Build history of the part. All positions in model axes, mm. A direction names the side the tool comes from. Coordinates: 2 decimals unless noted, no trailing zeros. Order: outer loops, then holes, each group sorted by start corner. A loop starts at its lowest first (then second) coordinate and runs counter-clockwise, first axis right, second up. Notation, with made-up numbers: (75.25, 17.25) - (123.25, 17.25) arc R19 ccw to (123.25, 43.25) - close; hole circle Ø10 at (57, 52). An arc over 180 degrees is marked (long way). Answer as CSV lines item,"result". Start each with the question number.
from build123d import *

# Parameters (mm, degrees)
SKETCH1_W                               = 96
SKETCH1_H                               = 64
BOSS_EXTRUDE1_DEPTH                     = 20
CBORE_FOR_M6_HEX_HEAD_BOLT1_D           = 6.4
CBORE_FOR_M6_HEX_HEAD_BOLT1_CBORE_D     = 14.547
CBORE_FOR_M6_HEX_HEAD_BOLT1_CBORE_DEPTH = 4
BOSS_EXTRUDE3_DEPTH                     = 60
CUT_EXTRUDE1_DEPTH                      = 12
SKETCH14_R                              = 26
SKETCH14_R_2                            = 16
BOSS_EXTRUDE4_DEPTH                     = 32
BOSS_EXTRUDE8_START                     = -12
BOSS_EXTRUDE8_DEPTH                     = 12
SKETCH17_R                              = 16
CUT_EXTRUDE2_DEPTH                      = 198.440406876


with BuildPart() as part:
    # Sketch1 → Boss-Extrude1 (new body)
    with BuildSketch(Plane(origin=(0, 0, 0), x_dir=(0, 0, -1), z_dir=(1, 0, 0))):
        Rectangle(SKETCH1_W, SKETCH1_H)
    extrude(amount=BOSS_EXTRUDE1_DEPTH)

    # CBORE for M6 Hex Head Bolt1 (through all)
    with Locations(Plane(origin=(20, 0, -30), x_dir=(0, 0, 1), z_dir=(1, 0, 0))):
        with Locations((0, 0)):
            cbore_for_m6_hex_head_bolt1 = CounterBoreHole(CBORE_FOR_M6_HEX_HEAD_BOLT1_D / 2, CBORE_FOR_M6_HEX_HEAD_BOLT1_CBORE_D / 2, CBORE_FOR_M6_HEX_HEAD_BOLT1_CBORE_DEPTH)

    # Mirror1: CBORE for M6 Hex Head Bolt1 across plane
    add(cbore_for_m6_hex_head_bolt1.mirror(Plane.XY), mode=Mode.SUBTRACT)

    # Sketch11 → Boss-Extrude3 (add)
    with BuildSketch(Plane(origin=(0, 0, -30), x_dir=(0, -1, 0), z_dir=(0, 0, 1))):
        with BuildLine():
            ThreePointArc((20, 97.56139982), (22.055252622, 107.893852494), (27.908116908, 116.653282912))
            Line((27.908116908, 116.653282912), (75.840620434, 164.585786438))
            Line((75.840620434, 164.585786438), (84.325901808, 156.100505063))
            Line((84.325901808, 156.100505063), (36.393398282, 108.168001538))
            ThreePointArc((36.393398282, 108.168001538), (33.141807012, 103.301651305), (32, 97.56139982))
            Line((32, 97.56139982), (32, 20))
            Line((32, 20), (20, 20))
            Line((20, 20), (20, 97.56139982))
        make_face()
    extrude(amount=BOSS_EXTRUDE3_DEPTH)

    # Sketch13 → Cut-Extrude1 (cut)
    with BuildSketch(Plane(origin=(44.372583002, 44.372583002, 0), x_dir=(0, 0, -1), z_dir=(0.7071067811865476, 0.7071067811865476, 0))):
        with BuildLine():
            Line((-30, -140.007142675), (-38.734920635, -140.007142675))
            Line((-38.734920635, -140.007142675), (-38.734920635, -179.207032884))
            Line((-38.734920635, -179.207032884), (30.889896781, -179.207032884))
            Line((30.889896781, -179.207032884), (30.889896781, -140.007142675))
            Line((30.889896781, -140.007142675), (30, -140.007142675))
            ThreePointArc((30, -140.007142675), (0, -170.007142675), (-30, -140.007142675))
        make_face()
    extrude(amount=-CUT_EXTRUDE1_DEPTH, mode=Mode.SUBTRACT)

    # Sketch14 → Boss-Extrude4 (add)
    with BuildSketch(Plane(origin=(44.372583002, 44.372583002, 0), x_dir=(0, 0, -1), z_dir=(0.7071067811865476, 0.7071067811865476, 0))):
        with Locations(Location((0, -140.007142675, 0), (0, 0, 90))):
            Circle(SKETCH14_R)
        with Locations(Location((0, -140.007142675, 0), (0, 0, 90))):
            Circle(SKETCH14_R_2, mode=Mode.SUBTRACT)
    extrude(amount=BOSS_EXTRUDE4_DEPTH)

    # Sketch16 → Boss-Extrude8 (add)
    with BuildSketch(Plane.XY.offset(6).offset(BOSS_EXTRUDE8_START)):
        with BuildLine():
            Line((20, 32), (20, -20))
            Line((20, -20), (97.56139982, -20))
            ThreePointArc((97.56139982, -20), (107.893852494, -22.055252622), (116.653282912, -27.908116908))
            Line((116.653282912, -27.908116908), (124.987806691, -36.242640687))
            Line((124.987806691, -36.242640687), (132.712452622, -43.967286618))
            Line((132.712452622, -43.967286618), (151.159621824, -25.520117415))
            Line((151.159621824, -25.520117415), (143.372583002, -17.857864376))
            Line((143.372583002, -17.857864376), (135.038059223, -9.523340597))
            ThreePointArc((135.038059223, -9.523340597), (117.843621735, 1.965615223), (97.56139982, 6))
            Line((97.56139982, 6), (55.38418899, 6))
            ThreePointArc((55.38418899, 6), (34.984926343, 15.315732711), (20, 32))
        make_face()
    extrude(amount=BOSS_EXTRUDE8_DEPTH)

    # Sketch17 → Cut-Extrude2 (cut, through all)
    with BuildSketch(Plane(origin=(67, 67, 0), x_dir=(0, 0, -1), z_dir=(0.7071067811865477, 0.7071067811865475, 0))):
        with Locations(Location((0, -140.007142675, 0), (0, 0, 90))):
            Circle(SKETCH17_R)
    extrude(amount=-CUT_EXTRUDE2_DEPTH, mode=Mode.SUBTRACT)


solid = part.part
(1) Probe L1, parallel to Y at x = 11, z = -30; L2, parallel to Z at x = 86, y = 0; L3, parallel to X at y = 1.5, z = 10.5. List the from-to ranges inside material, lowest first. Write a range as [from, to].
(2) Band-saw the part on A-A on y = 0. List the corners of the cut face in (x, z), plus the area to 3 significant figures.
(3) Pull direction Y, two halves, no side cores. Call faces 1 (the flat face through (58, -20, 18)), 2 (the flat face through (10, 0, 48)), 3 (the cylindrical face through (103.378, -33.174, -0.42)), 4 (the cylindrical face through (7.9, -0.1, -26.8)): +Y half, -Y half, draft (parallel to the pull), parting line (faces both ways), or undercut.
(4) Which spindle directions (+Z, -Z, +X, -X, +Y, -Y) get a long thin tool onto all of the face, cutting with end or side? Do faces 5 (the cylindrical face through (107.76, -22, -18.17)), 6 (the cylindrical face through (107.76, -22, 17.83)), 7 (the flat face through (139.264, -13.749, -0.084)), 8 (the flat face through (16, 2, 27)), 9 (the flat face through (37, -32, 1)). Say none if no direction does.
(5) Band-saw the part on B-B on x = 82. List the corners of the cut face in (y, z).
(6) Drop flat-ended pins along their axis: pin 1 Ø12.5 at (y, z) = (7, -26) entering from +X; pin 2 Ø8 at (x, z) = (25, -22.5) entering from +Y; pin 3 Ø2 at (x, z) = (38.5, -32) entering from -Y; pin 4 Ø10 at (x, y) = (136, -33) entering from -Z. Give the stop position or say it passes through.
Filled in:
1,L1,"y = [-32, -3.2], [3.2, 32]"
1,L2,"z = [-6, 6]"
1,L3,"x = [0, 20]"
2,outline,"(0, -48) - (20, -48) - (20, -37.27) - (16, -37.27) - (16, -33.2) - (0, -33.2) - close; (0, -26.8) - (16, -26.8) - (16, -22.73) - (20, -22.73) - (20, -6) - (122.06, -6) - (122.06, 6) - (20, 6) - (20, 22.73) - (16, 22.73) - (16, 26.8) - (0, 26.8) - close; (0, 33.2) - (16, 33.2) - (16, 37.27) - (20, 37.27) - (20, 48) - (0, 48) - close"
2,area,"2,820 mm^2"
3,face 1,"+Y half"
3,face 2,"draft"
3,face 3,"-Y half"
3,face 4,"undercut"
4,face 5,"-Z, +Y"
4,face 6,"+Z, +Y"
4,face 7,"+Z, -Z, +Y"
4,face 8,"+X"
4,face 9,"+Z, -Z, -X, -Y"
5,outline,"(-32, -30) - (-20, -30) - (-20, -6) - (6, -6) - (6, 6) - (-20, 6) - (-20, 30) - (-32, 30) - close"
6,pin 1,"stops at x = 20"
6,pin 2,"stops at y = -20"
6,pin 3,"passes through"
6,pin 4,"stops at z = -20.87"
